The figure shows three views and two pictorial views of one solid part (mm, origin at its lowest corner). Answer the questions. Give positions to 0.01 mm unless a question says otherwise; leave off trailing zeros. Write each loop counter-clockwise with the first axis right and the second up, starting at its lowest first coordinate (ties: lowest second). Pieces come first, ordered by that corner, then holes. Notation, with made-up numbers: (87.5, -32.75) -> (92.5, -32.75) arc R27 cw to (92.5, -13.75) -> close; hole circle Ø3 at (76.5, -6.5). An arc over 180 degrees is marked (long way). Write item = value, one per line. Start each with the question number.
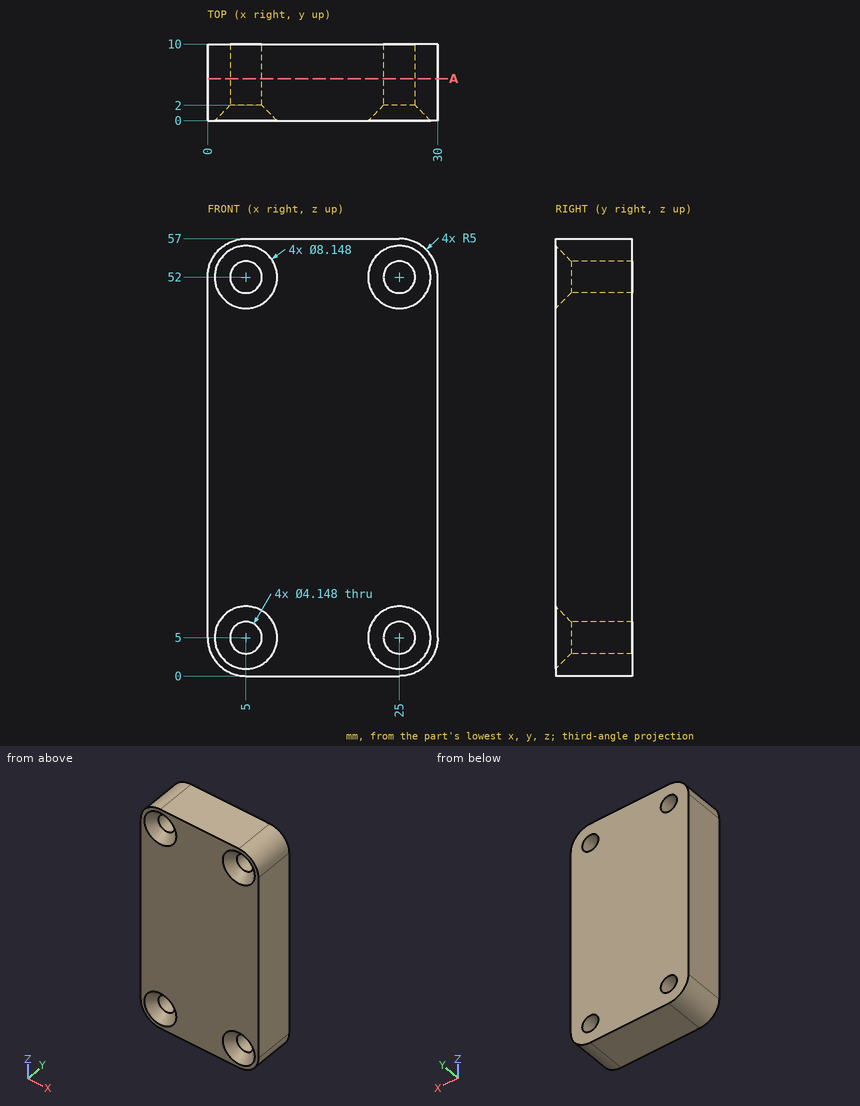
(1) Find the intervals of material crossed by line 1 along Z through (x, y) = (25, 6.5); line 2 along Z through (x, y) = (25.5, 4.5); line 3 along Y through (x, z) = (28, 2.5), in increasing order.
(2) A cutting plane is placed at A-A, the plane y = 5.5. Write down the section's boundary in (x, z).
(3) Each of these flat-tipped pins is pushed along its axis until it touches: pin 1 (6.5 mm diameter, centred on x = 5, z = 52, fed in from -Y); pin 2 (2.5 mm diameter, centred on x = 5, z = 5, fed in from -Y); pin 3 (1 mm diameter, centred on x = 3.5, y = 2, fed in from +Z); pin 4 (5 mm diameter, centred on x = 25, z = 5, fed in from -Y). Where does it stop, or does it pass through?
Results list:
q1.line_1 = 0 to 2.93, 7.07 to 49.93, 54.07 to 57
q1.line_2 = 0.03 to 2.99, 7.01 to 49.99, 54.01 to 56.97
q1.line_3 = 0.17 to 10
q2.outline = (0, 5) arc R5 ccw to (5, 0) -> (25, 0) arc R5 ccw to (30, 5) -> (30, 52) arc R5 ccw to (25, 57) -> (5, 57) arc R5 ccw to (0, 52) -> close; hole circle Ø4.15 at (5, 5); hole circle Ø4.15 at (5, 52); hole circle Ø4.15 at (25, 5); hole circle Ø4.15 at (25, 52)
q3.pin_1 = 0.82
q3.pin_2 = through
q3.pin_3 = 56.9
q3.pin_4 = 1.57
